The listing builds one solid part. Answer for the finished solid, in the listing's coordinates (mm). A direction names the side the tool comes from. Coordinates: 2 decimals unless noted, no trailing zeros. Order: outer loops, then holes, each group sorted by start corner. A loop starts at its lowest first (then second) coordinate and runs counter-clockwise, first axis right, second up. Notation, with made-up numbers: (-18.5, -31.75) -> (21.5, -31.75) arc R27 ccw to (21.5, -5.75) -> close; hole circle Ø4 at (27.25, 61). An arc over 180 degrees is marked (long way). Put each result on its own line as item: value. Start each with the question number.
```python
from build123d import *

# Parameters (mm, degrees)
F0_W     = 16.7894
F0_H     = 23.749
F1_DEPTH = 12.8778
F2_R     = 0.5
F4_DEPTH = 10
F5_R     = 1.5875
F6_DEPTH = 0.9906
F7_W     = 0.6096
F7_H     = 1.397
F8_DEPTH = 0.254
F9_SIZE  = 0.381


with BuildPart() as f1:
    # F0 (on Top) → F1 (new body)
    with BuildSketch(Plane.XY):
        Rectangle(F0_W, F0_H)
    extrude(amount=F1_DEPTH)

    # F2
    f2_edges = [f1.edges().sort_by_distance(p)[0] for p in [
        (8.3947, 11.8745, 6.4389),
        (-8.3947, 11.8745, 6.4389),
        (0, -11.8745, 12.8778),
        (-8.3947, 0, 12.8778),
        (0, 11.8745, 12.8778),
        (8.3947, 0, 12.8778),
        (-8.3947, -11.8745, 6.4389),
        (8.3947, -11.8745, 6.4389),
    ]]
    fillet(f2_edges, radius=F2_R)

    # F3 (on face) → F4 (cut)
    with BuildSketch(Plane.XZ.offset(11.8745)):
        Polygon((6.5885786898, 10.8017679304), (0, 10.8017679304), (-6.5885786898, 10.8017679304), (-6.5885786898, 3.4128425177), (-4.8500075936, 3.4128425177), (-4.8500075936, 1.597570139), (-3.7250500172, 1.597570139), (-3.7250500172, 0.6771502085), (0, 0.6771502085), (3.7250500172, 0.6771502085), (3.7250500172, 1.597570139), (4.8500075936, 1.597570139), (4.8500075936, 3.4128425177), (6.5885786898, 3.4128425177), align=None)
    extrude(amount=-F4_DEPTH, mode=Mode.SUBTRACT)

    # F5 (on face) → F6 (join)
    with BuildSketch(Plane(origin=(0, 0, 0), x_dir=(1, 0, 0), z_dir=(0, 0, -1))):
        with Locations((6.35, 0.9525)):
            Circle(F5_R)
        with Locations((-6.35, 0.9525)):
            Circle(F5_R)
    extrude(amount=F6_DEPTH)

    # F7 (on face) → F8 (join)
    with BuildSketch(Plane(origin=(0, 0, 0), x_dir=(1, 0, 0), z_dir=(0, 0, -1))):
        with Locations((1.016, -12.5095)):
            Rectangle(F7_W, F7_H)
        with Locations((3.048, -12.5095)):
            Rectangle(F7_W, F7_H)
        with Locations((5.08, -12.5095)):
            Rectangle(F7_W, F7_H)
        with Locations((-1.016, -12.5095)):
            Rectangle(F7_W, F7_H)
        with Locations((-5.08, -12.5095)):
            Rectangle(F7_W, F7_H)
        with Locations((-3.048, -12.5095)):
            Rectangle(F7_W, F7_H)
        with BuildLine():
            Line((9.1567, 4.5085), (8.3947, 4.5085))
            Line((8.3947, 4.5085), (8.3947, 2.4765))
            Line((8.3947, 2.4765), (9.1567, 2.4765))
            ThreePointArc((9.1567, 2.4765), (9.3363051224, 2.5508948776), (9.4107, 2.7305))
            Line((9.4107, 2.7305), (9.4107, 4.2545))
            ThreePointArc((9.4107, 4.2545), (9.3363051224, 4.4341051224), (9.1567, 4.5085))
        make_face()
        with BuildLine():
            ThreePointArc((-9.1567, 4.5085), (-9.3363051224, 4.4341051224), (-9.4107, 4.2545))
            Line((-9.4107, 4.2545), (-9.4107, 2.7305))
            ThreePointArc((-9.4107, 2.7305), (-9.3363051224, 2.5508948776), (-9.1567, 2.4765))
            Line((-9.1567, 2.4765), (-8.3947, 2.4765))
            Line((-8.3947, 2.4765), (-8.3947, 4.5085))
            Line((-8.3947, 4.5085), (-9.1567, 4.5085))
        make_face()
    extrude(amount=-F8_DEPTH)

    # F9
    f9_edges = [f1.edges().sort_by_distance(p)[0] for p in [
        (4.7625, -0.9525, -0.9906),
        (-7.9375, -0.9525, -0.9906),
    ]]
    chamfer(f9_edges, length=F9_SIZE)


solid = f1.part
```
(1) A tool of negligible diameter and unlimited length cuts with its end or side. For faces 3 (the cylindrical face through (-5.617, 0.456, -0.301)), 4 (the flat face through (-9, -4, 0.254)), 5 (the flat face through (-6.589, -7, 7)), from which of +Z, -Z, +X, -X, +Y, -Y can it reach the whole face along a straight path? Write none if from no direction.
(2) The part is cut by section D-D on z = 11.25. Determine the outline of the cut face in (x, y).
(3) Each of these flat-tipped pins is pushed along its axis until it touches: P1, Ø0.7, axis at x = -5, y = 12.5, coming from the +Z side; P2, Ø3, axis at x = 0, z = 4.5, coming from the +Y side; P3, Ø1, axis at y = 9.5, z = 7, coming from the +X side. Where does it stop, or does it pass through?
(4) The part is cut by section C-C on z = 2. Determine the outline of the cut face in (x, y), plus the area to 3 significant figures.
(5) Find the intervals of material crossed by L1, parallel to X at y = -5, z = 8; L2, parallel to X at y = -10.75, z = 1; L3, parallel to Z at x = 5.5, y = -8.5, in increasing order.
(6) The part is cut by section B-B on y = 2.25. Determine the outline of the cut face in (x, z), plus the area to 3 significant figures.
(7) The part is cut by section A-A on z = 3.75. Determine the outline of the cut face in (x, y), plus the area to 3 significant figures.
(8) For a pull along X with two mould halves and no side action, classify faces 1 (the flat face through (-6, -7, 3.413)), 2 (the flat face through (0, 0, 12.878)) as released by +X, released by -X, zero draft, split by the parting line, or undercut.
Worked out:
1. face 3: -Z
1. face 4: +Z, -X, +Y, -Y
1. face 5: -Y
2. outline: (-8.39, -11.37) arc R0.5 ccw to (-7.89, -11.87) -> (7.89, -11.87) arc R0.5 ccw to (8.39, -11.37) -> (8.39, 11.37) arc R0.5 ccw to (7.89, 11.87) -> (-7.89, 11.87) arc R0.5 ccw to (-8.39, 11.37) -> close
3. P1: z = 0.25
3. P2: y = 11.87
3. P3: x = 8.39
4. outline: (-8.39, -11.37) arc R0.5 ccw to (-7.89, -11.87) -> (-4.85, -11.87) -> (-4.85, -1.87) -> (4.85, -1.87) -> (4.85, -11.87) -> (7.89, -11.87) arc R0.5 ccw to (8.39, -11.37) -> (8.39, 11.37) arc R0.5 ccw to (7.89, 11.87) -> (-7.89, 11.87) arc R0.5 ccw to (-8.39, 11.37) -> close
4. area: 302 mm2
5. L1: -8.39 to -6.59, 6.59 to 8.39
5. L2: -8.39 to -3.73, 3.73 to 8.39
5. L3: 0 to 3.41, 10.8 to 12.88
6. outline: (-8.39, 0) -> (8.39, 0) -> (8.39, 12.38) arc R0.5 ccw to (7.89, 12.88) -> (-7.89, 12.88) arc R0.5 ccw to (-8.39, 12.38) -> close
6. area: 216 mm2
7. outline: (-8.39, -11.37) arc R0.5 ccw to (-7.89, -11.87) -> (-6.59, -11.87) -> (-6.59, -1.87) -> (6.59, -1.87) -> (6.59, -11.87) -> (7.89, -11.87) arc R0.5 ccw to (8.39, -11.37) -> (8.39, 11.37) arc R0.5 ccw to (7.89, 11.87) -> (-7.89, 11.87) arc R0.5 ccw to (-8.39, 11.37) -> close
7. area: 267 mm2
8. face 1: undercut
8. face 2: zero draft
